Design review of the part shown in the three views and the two pictorial views. Dimensions are in mm from the part's minimum x, y and z. Coordinates: 2 decimals unless noted, no trailing zeros. Write each loop counter-clockwise with the first axis right and the second up, starting at its lowest first coordinate (ties: lowest second). Pieces come first, ordered by that corner, then holes. Notation, with made-up numbers: (8.25, 89) - (39.25, 89) arc R25 ccw to (39.25, 112) - close; hole circle Ø1 at (20, 51). An arc over 180 degrees is marked (long way). Return JSON: item names as keys, results as strings. Group by question number.
(1) We need section D-D on z = 24.5. State the section outline as (x, y) points, then the cut area to 3 significant figures.
(2) We need section B-B on z = 2.25. State the section outline as (x, y) points, then the cut area to 3 significant figures.
(3) We need section A-A on y = 2.7. State the section outline as (x, z) points, then the cut area to 3 significant figures.
(4) For pin 1 Ø1.1 at (x, y) = (11.5, 0.5) entering from +Z, flat-tipped, find the tip position at first contact; note if it passes through.
(5) We need section C-C on x = 4.25. State the section outline as (y, z) points.
(6) To check wall thickness, follow L1, parallel to X at y = 2.55, z = 2.25; L2, parallel to Y at x = 13.75, z = 22; L3, parallel to Z at x = 4.25, y = 0.85. State the ranges of each line that lie inside material, in increasing order. Write a range as from..to.
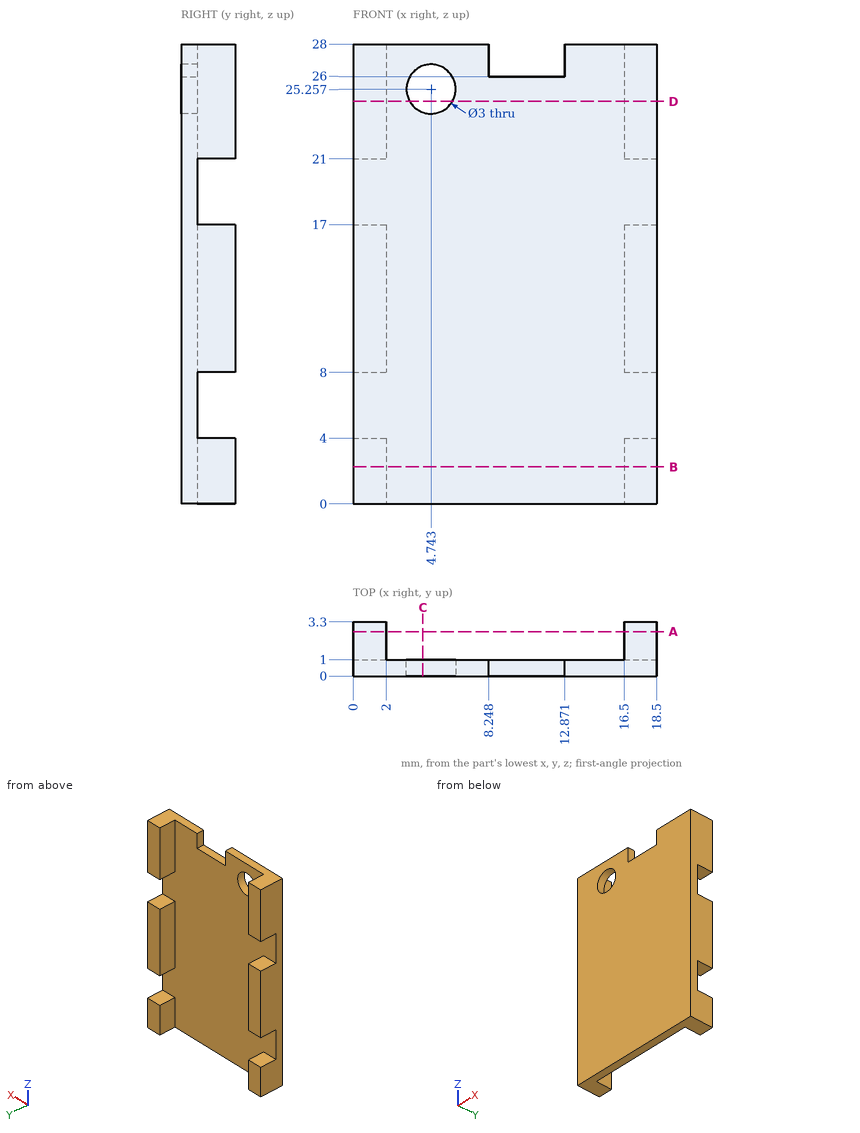
Ans:
{
 "1": {"outline": "(0, 0) - (3.45, 0) - (3.45, 1) - (2, 1) - (2, 3.3) - (0, 3.3) - close; (6.04, 0) - (18.5, 0) - (18.5, 3.3) - (16.5, 3.3) - (16.5, 1) - (6.04, 1) - close", "area": "25.1 mm²"},
 "2": {"outline": "(0, 0) - (18.5, 0) - (18.5, 3.3) - (16.5, 3.3) - (16.5, 1) - (2, 1) - (2, 3.3) - (0, 3.3) - close", "area": "27.7 mm²"},
 "3": {"outline": "(0, 0) - (2, 0) - (2, 4) - (0, 4) - close; (0, 8) - (2, 8) - (2, 17) - (0, 17) - close; (0, 21) - (2, 21) - (2, 28) - (0, 28) - close; (16.5, 0) - (18.5, 0) - (18.5, 4) - (16.5, 4) - close; (16.5, 8) - (18.5, 8) - (18.5, 17) - (16.5, 17) - close; (16.5, 21) - (18.5, 21) - (18.5, 28) - (16.5, 28) - close", "area": "80.0 mm²"},
 "4": {"pin 1": "z = 26"},
 "5": {"outline": "(0, 0) - (1, 0) - (1, 23.84) - (0, 23.84) - close; (0, 26.67) - (1, 26.67) - (1, 28) - (0, 28) - close"},
 "6": {"L1": "0..2, 16.5..18.5", "L2": "0..1", "L3": "0..23.84, 26.67..28"}
}
